Geometry: final body of the model. Coordinates: model frame, mm. A direction names the side the tool comes from. Coordinates: 2 decimals unless noted, no trailing zeros. Loops run counter-clockwise (first coordinate to the right, second up) from the corner with the lowest first, then second, coordinate; pieces in that order, holes last. Notation, with made-up numbers: (-18, -1.75) - (36, -1.75) arc R23 cw to (36, 27.25) - close; hole circle Ø10 at (-11, 47.5). An arc over 180 degrees is marked (long way). Put each result on its own line as item: value. Start each with the question number.
1) Material intervals for line 1 along X through (y, z) = (-7, 5); line 2 along Z through (x, y) = (11, -2); line 3 along X through (y, z) = (-7, 8), sorted ascending. Write a range as from..to.
2) Section D-D on z = 5.5. Output: boundary loops of the cut face in (x, y), and give its area (3 significant figures).
3) Section A-A on z = 9. Output: boundary loops of the cut face in (x, y), and give its area (3 significant figures).
4) Draft query along Y for faces 1 (the cylindrical face through (4.737, -7.676, 5.316)), 2 (the flat face through (15, -3, 9)), 3 (the cylindrical face through (11, -2, 10)). Return one class per face: +Y half, -Y half, draft (parallel to the pull), parting line (faces both ways), or undercut.
5) Contact query for flat-ended pins moving along their axis: pin 1 Ø3.5 at (x, y) = (11.5, -7.5) entering from +Z; pin 2 Ø3 at (y, z) = (-18.5, 9) entering from +X; pin 3 Ø1.6 at (x, y) = (4, -6.5) entering from +Z. Output: stop coordinate, or through.
6) Reachability of faces 4 (the flat face through (8, -7, 8)), 5 (the flat face through (8, 0, 6)), 6 (the flat face through (3, -10, 10)), 7 (the flat face through (4, -7, 0.5)) from +Z, -Z, +X, -X, +Y, -Y: full face, straight path, thin tool, end or side. Return the list, or none.
7) Section B-B on y = -7. Output: boundary loops of the cut face in (x, z).
8) Section C-C on x = 6.5. Output: boundary loops of the cut face in (y, z), and give its area (3 significant figures).
Autodesk Fusion 360 part; units mm, degrees
sketch "Sketch1" plane through (0, 0, 0) normal (0, 0, 1) x (1, 0, 0)
  line L0 (0, 0) -> (16, 0)
  line L1 (16, 0) -> (16, -14)
  line L2 (0, -20) -> (10, -20)
  line L3 (0, -20) -> (0, 0)
  line L4 (10, -20) -> (16, -14)
  dimension "d1" = 16
  dimension "d2" = 14
  dimension "d3" = 10
  dimension "d4" = 20
extrude "Extrude1" add sketch "Sketch1" along normal blind 6
sketch "Sketch2" plane through (0, 0, 6) normal (0, 0, 1) x (-1, 0, 0)
  line L0 (0, 20) -> (-10, 20)
  line L1 (-10, 20) -> (-16, 14)
  line L2 (-16, 14) -> (-16, 0)
  line L3 (-16, 0) -> (0, 0)
  line L4 (0, 0) -> (0, 20)
  line L5 (0, 0) -> (-14, 0)
  line L6 (-14, 0) -> (-14, 4)
  line L7 (-14, 4) -> (0, 4)
  line L8 (0, 4) -> (0, 0)
  line L9 (-14, 4) -> (-16, 2)
  line L10 (-14, 4) -> (-11.1716, 4) construction
  line L11 (0, 20) -> (-4, 20)
  line L12 (-4, 20) -> (-4, 4)
  line L13 (-4, 4) -> (0, 4)
  line L14 (0, 4) -> (0, 20)
  line L15 (0, 4) -> (-8, 4)
  line L16 (-8, 4) -> (-8, 10)
  line L17 (-8, 10) -> (0, 10)
  line L18 (0, 10) -> (0, 4)
  line L19 (-8, 10) -> (-4, 16)
  dimension "d7" = 14
  dimension "d8" = 4
  dimension "d9" = 135
  dimension "d10" = 4
  dimension "d11" = 8
  dimension "d12" = 6
  dimension "d13" = 4
extrude "Extrude2" add sketch "Sketch2" along normal blind 4 contours L0 L4 L11 L12 L14 L17 | L4 L7 L12 L13 L14 L15 L17 L18 | L12 L17 L19 | L7 L12 L15 L16 L17
extrude "Extrude3" add sketch "Sketch2" along normal blind 6 contours L3 L4 L5 L6 L7 L8 L13 L15 | L2 L3 L6 L9
sketch "Sketch3" plane through (0, -4, 0) normal (0, -1, 0) x (1, 0, 0)
  line L0 (0, 10) -> (8, 10)
  line L1 (8, 10) -> (8, 6)
  line L2 (8, 6) -> (14, 6)
  line L3 (14, 6) -> (14, 12)
  line L4 (14, 12) -> (0, 12)
  line L5 (0, 12) -> (0, 10)
  circle A0 centre (11, 9) radius 1
  dimension "d18" = 2
  dimension "d19" = 3
  dimension "d20" = 3
extrude "Extrude4" cut sketch "Sketch3" against normal blind 9 contours A0
sketch "Sketch4" plane through (0, 0, 10) normal (0, 0, 1) x (-1, 0, 0)
  line L0 (0, 4) -> (0, 20)
  line L1 (0, 20) -> (-4, 20)
  line L2 (-4, 20) -> (-4, 16)
  line L3 (-4, 16) -> (-8, 10)
  line L4 (-8, 10) -> (-8, 4)
  line L5 (-8, 4) -> (0, 4)
  circle A0 centre (-4, 7) radius 1
  dimension "d23" = 2
  dimension "d24" = 4
  dimension "d25" = 3
extrude "Extrude5" cut sketch "Sketch4" against normal blind 9.5 contours A0
Answer block:
1. line 1: x = 0..3, 5..16
1. line 2: z = 0..8, 10..12
1. line 3: x = 0..3, 5..8
2. outline: (0, -20) - (10, -20) - (16, -14) - (16, 0) - (0, 0) - close; hole circle Ø2 at (4, -7)
2. area: 299 mm²
3. outline: (0, -20) - (4, -20) - (4, -16) - (8, -10) - (8, -4) - (10, -4) - (10, 0) - (0, 0) - close; (12, -4) - (14, -4) - (16, -2) - (16, 0) - (12, 0) - close; hole circle Ø2 at (4, -7)
3. area: 151 mm²
4. face 1: undercut
4. face 2: -Y half
4. face 3: draft
5. pin 1: stops at z = 6
5. pin 2: stops at x = 4
5. pin 3: stops at z = 10
6. face 4: +Z, +X, -Y
6. face 5: +Z, -Z, +X, -X, +Y
6. face 6: +Z, +X, -X, -Y
6. face 7: +Z
7. outline: (0, 0) - (16, 0) - (16, 6) - (8, 6) - (8, 10) - (5, 10) - (5, 0.5) - (3, 0.5) - (3, 10) - (0, 10) - close
8. outline: (-20, 0) - (0, 0) - (0, 12) - (-4, 12) - (-4, 10) - (-12.25, 10) - (-12.25, 6) - (-20, 6) - close
8. area: 177 mm²
